Source: CAD feature listing. Evaluate the final solid. Frame: model axes, mm. Face numbers are marked on the shaded views. A direction names the side the tool comes from. Round coordinates to 2 decimals unless told otherwise and drop trailing zeros. Loops run counter-clockwise (first coordinate to the right, second up) from the corner with the lowest first, then second, coordinate; pieces in that order, holes last.
(1) Section D-D, the plane z = -21. Return the cut outline in (x, y) (3 decimals), plus the area to 3 significant figures.
(2) Section C-C, the plane y = 57.5. Return the cut outline in (x, z) (3 decimals).
(3) Mould query, pull axis X, two halves, no side actions, for the marked faces 4, 5, 6 and 7. Classes: pulls with the +X half, pulls with the -X half, needs draft (parallel to the pull), parting line crosses it, or undercut.
(4) Set-up query: the marked faces 1, 2 and 3. Return all of +Z, -Z, +X, -X, +Y, -Y with unobstructed straight access to the full face (end or side cutting, diameter ignored); none if empty.
(5) Section B-B, the plane z = 0. Return the cut outline in (x, y) (3 decimals), plus the area to 3 significant figures.
(6) Material intervals for probe 1 along X at (y, z) = (66.95, -37) (3 decimals); probe 2 along Z at (x, y) = (64.5, 15); probe 3 along Z at (x, y) = (-18, 11.5) (3 decimals), sorted ascending.
(7) First-contact query: pin 1 Ø6.5 at (y, z) = (11.5, 3) entering from +X; pin 2 Ø1.5 at (x, y) = (-18, 13) entering from -Z; pin 3 Ø1.5 at (x, z) = (18, -8) entering from -Y; pin 4 Ø1.5 at (x, z) = (-11.5, -9) entering from +Y. Flat tips, straight axial feed; report the tip coordinate or a pass-through.
(8) Section A-A, the plane x = 1.5. Return the cut outline in (y, z) (3 decimals), plus the area to 3 significant figures.
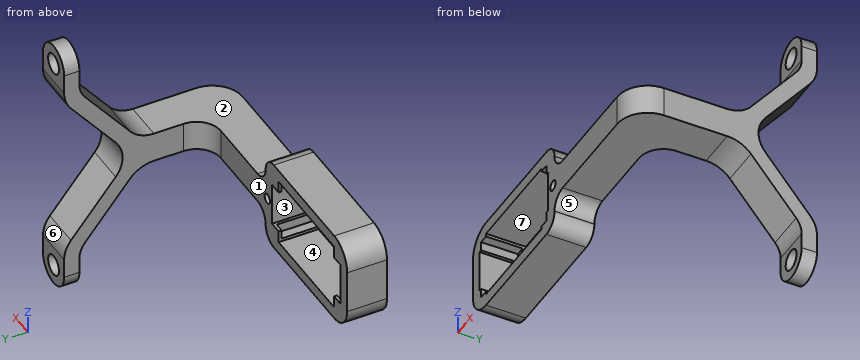
```python
from build123d import *

# Parameters (mm, degrees)
BOSS_EXTRUDE1_DEPTH                   = 1
BOSS_EXTRUDE1_DEPTH_BACK              = 12
SKETCH1_W                             = 50.25
SKETCH1_H                             = 30.25
BOSS_EXTRUDE2_DEPTH                   = 5
BOSS_EXTRUDE3_DEPTH                   = 5
SKETCH4_R                             = 3.35
CUT_EXTRUDE1_DEPTH                    = 10
SKETCH6_W                             = 4
SKETCH6_H                             = 4
BOSS_EXTRUDE4_DEPTH                   = 1
TAP_DRILL_FOR_M4X0_7_TAP1_D           = 3.3
TAP_DRILL_FOR_M4X0_7_TAP1_CSINK_D     = 3.35
TAP_DRILL_FOR_M4X0_7_TAP1_CSINK_ANGLE = 90
SKETCH13_W                            = 13
SKETCH13_H                            = 54
CUT_EXTRUDE2_DEPTH                    = 22
BOSS_EXTRUDE5_DEPTH                   = 13
FILLET1_R                             = 10
FILLET2_R                             = 8
FILLET3_R                             = 5
FILLET4_R                             = 8


with BuildPart() as part:
    # Sketch1 → Boss-Extrude1 (new, two sides: drawn at the far end of the back side and taken through both)
    with BuildSketch(Plane(origin=(0, 20.13, 0), x_dir=(1, 0, 0), z_dir=(0, 1, 0)).offset(-BOSS_EXTRUDE1_DEPTH_BACK)):
        Rectangle(SKETCH1_W, SKETCH1_H)
        Polygon((20.125, 10.125), (17.125, 10.125), (17.125, 11.125), (-17.125, 11.125), (-17.125, 10.125), (-20.125, 10.125), (-20.125, 7.125), (-21.125, 7.125), (-21.125, -7.125), (-20.125, -7.125), (-20.125, -10.125), (-17.125, -10.125), (-17.125, -11.125), (17.125, -11.125), (17.125, -10.125), (20.125, -10.125), (20.125, -7.125), (21.125, -7.125), (21.125, 7.125), (20.125, 7.125), align=None, mode=Mode.SUBTRACT)
    extrude(amount=BOSS_EXTRUDE1_DEPTH + BOSS_EXTRUDE1_DEPTH_BACK)

    # Sketch2 → Boss-Extrude2 (add, symmetric)
    with BuildSketch(Plane.XY):
        Polygon((25.125, 21.13), (60.625, 21.13), (60.625, 68.13), (73.625, 68.13), (73.625, 8.13), (25.125, 8.13), align=None)
    extrude(amount=BOSS_EXTRUDE2_DEPTH, both=True)

    # Sketch3 → Boss-Extrude3 (add)
    with BuildSketch(Plane(origin=(0, 68.13, 0), x_dir=(1, 0, 0), z_dir=(0, 1, 0))):
        with BuildLine():
            Line((73.625, 5), (73.625, 37))
            ThreePointArc((73.625, 37), (67.125, 43.5), (60.625, 37))
            Line((60.625, 37), (60.625, 5))
            Line((60.625, 5), (73.625, 5))
        make_face()
        with BuildLine():
            Line((73.625, -37), (73.625, -5))
            Line((73.625, -5), (60.625, -5))
            Line((60.625, -5), (60.625, -37))
            ThreePointArc((60.625, -37), (67.125, -43.5), (73.625, -37))
        make_face()
    extrude(amount=-BOSS_EXTRUDE3_DEPTH)

    # Sketch4 → Cut-Extrude1 (cut)
    with BuildSketch(Plane.XZ.offset(-63.13)):
        with Locations(Location((67.125, 37, 0), (0, 0, 270))):
            Circle(SKETCH4_R)
        with Locations(Location((67.125, -37, 0), (0, 0, 270))):
            Circle(SKETCH4_R)
    extrude(amount=-CUT_EXTRUDE1_DEPTH, mode=Mode.SUBTRACT)

    # Sketch6 → Boss-Extrude4 (add)
    with BuildSketch(Plane(origin=(0, 21.13, 0), x_dir=(1, 0, 0), z_dir=(0, 1, 0))):
        with Locations((19.125, 9.125)):
            Rectangle(SKETCH6_W, SKETCH6_H)
        with Locations((19.125, -9.125)):
            Rectangle(SKETCH6_W, SKETCH6_H)
        with Locations((-19.125, -9.125)):
            Rectangle(SKETCH6_W, SKETCH6_H)
        with Locations((-19.125, 9.125)):
            Rectangle(SKETCH6_W, SKETCH6_H)
    extrude(amount=-BOSS_EXTRUDE4_DEPTH)

    # Tap Drill for M4x0.7 Tap1 (through all)
    with Locations(Plane(origin=(0, 8.13, 0), x_dir=(-1, 0, 0), z_dir=(0, -1, 0))):
        with Locations((-24.125, 0)):
            CounterSinkHole(TAP_DRILL_FOR_M4X0_7_TAP1_D / 2, TAP_DRILL_FOR_M4X0_7_TAP1_CSINK_D / 2, counter_sink_angle=TAP_DRILL_FOR_M4X0_7_TAP1_CSINK_ANGLE)

    # Sketch13 → Cut-Extrude2 (cut)
    with BuildSketch(Plane(origin=(0, 68.13, 0), x_dir=(1, 0, 0), z_dir=(0, 1, 0))):
        with Locations((67.125, 0)):
            Rectangle(SKETCH13_W, SKETCH13_H)
    extrude(amount=-CUT_EXTRUDE2_DEPTH, mode=Mode.SUBTRACT)


with BuildPart() as cut_extrude2_piece_1:
    # of the separate pieces the step leaves, piece 1, a body of its own (cut_extrude2_pieces)
    add(part.part.solids().sort_by_distance((25.125, 21.13, 15.125))[0])



with BuildPart() as cut_extrude2_piece_2:
    # of the separate pieces the step leaves, piece 2, a body of its own (cut_extrude2_pieces)
    add(part.part.solids().sort_by_distance((73.625, 68.13, 27))[0])


with BuildPart() as cut_extrude2_piece_3:
    # of the separate pieces the step leaves, piece 3, a body of its own (cut_extrude2_pieces)
    add(part.part.solids().sort_by_distance((73.625, 63.13, -27))[0])


with BuildPart() as cut_extrude2_piece_1_1:
    add(cut_extrude2_piece_1.part)

    add(cut_extrude2_piece_2.part)  # Boss-Extrude5 merges Cut-Extrude2 piece 2

    add(cut_extrude2_piece_3.part)  # Boss-Extrude5 merges Cut-Extrude2 piece 3
    # Sketch14 → Boss-Extrude5 (add)
    with BuildSketch(Plane(origin=(73.625, 0, 0), x_dir=(0, 0, -1), z_dir=(1, 0, 0))):
        Polygon((29, 63.13), (27, 63.13), (27, 68.13), (0, 46.13), (5, 46.13), (5, 43.574444444), align=None)
        Polygon((-5, 46.13), (0, 46.13), (-27, 68.13), (-27, 63.13), (-29, 63.13), (-5, 43.574444444), align=None)
    extrude(amount=-BOSS_EXTRUDE5_DEPTH)

    # Fillet1
    fillet1_edges = [cut_extrude2_piece_1_1.edges().sort_by_distance(p)[0] for p in [
        (73.625, 8.13, 0),
        (67.125, 43.574444444, -5),
        (67.125, 46.13, 0),
        (67.125, 68.13, -27),
        (67.125, 43.574444444, 5),
        (67.125, 68.13, 27),
    ]]
    fillet(fillet1_edges, radius=FILLET1_R)

    # Fillet2
    fillet2_edges = [cut_extrude2_piece_1_1.edges().sort_by_distance(p)[0] for p in [
        (67.125, 63.13, -29),
        (67.125, 63.13, 29),
    ]]
    fillet(fillet2_edges, radius=FILLET2_R)

    # Fillet3
    fillet3_edges = [cut_extrude2_piece_1_1.edges().sort_by_distance(p)[0] for p in [
        (25.125, 14.63, 5),
        (25.125, 14.63, 15.125),
        (25.125, 14.63, -5),
        (25.125, 14.63, -15.125),
    ]]
    fillet(fillet3_edges, radius=FILLET3_R)

    # Fillet4
    fillet4_edges = [cut_extrude2_piece_1_1.edges().sort_by_distance(p)[0] for p in [
        (60.625, 21.13, 0),
        (-25.125, 14.63, 15.125),
        (-25.125, 14.63, -15.125),
    ]]
    fillet(fillet4_edges, radius=FILLET4_R)


solid = cut_extrude2_piece_1_1.part
```
Output values:
1. outline: (60.625, 56.611) - (73.625, 56.611) - (73.625, 63.241) - (60.625, 63.241) - close
1. area: 86.2 mm2
2. outline: (60.625, -22.09) - (73.625, -22.09) - (73.625, -13.954) - (60.625, -13.954) - close; (60.625, 13.954) - (73.625, 13.954) - (73.625, 22.09) - (60.625, 22.09) - close
3. face 4: undercut
3. face 5: pulls with the +X half
3. face 6: needs draft
3. face 7: undercut
4. face 1: +Z, -Z, -X, +Y
4. face 2: +Z, +X, -Y
4. face 3: +Y, -Y
5. outline: (-25.125, 8.13) - (-21.125, 8.13) - (-21.125, 21.13) - (-25.125, 21.13) - close; (21.125, 8.13) - (22.45, 8.13) - (22.475, 8.155) - (22.475, 21.13) - (21.125, 21.13) - close; (25.775, 8.155) - (25.8, 8.13) - (63.625, 8.13) arc R10 ccw to (73.625, 18.13) - (73.625, 49.029) - (60.625, 49.029) - (60.625, 29.13) arc R8 cw to (52.625, 21.13) - (25.775, 21.13) - close
5. area: 1,050 mm2
6. probe 1: x = 60.625 to 63.775, 70.475 to 73.625
6. probe 2: z = -5 to 5
6. probe 3: z = -15.077 to -10.125, 10.125 to 15.077
7. pin 1: stops at x = 73.04
7. pin 2: stops at z = -15.12
7. pin 3: stops at y = 20.13
7. pin 4: passes through
8. outline: (8.13, -15.125) - (21.13, -15.125) - (21.13, -11.125) - (8.13, -11.125) - close; (8.13, 11.125) - (21.13, 11.125) - (21.13, 15.125) - (8.13, 15.125) - close
8. area: 104 mm2
